Design review of the part built by this model. Coordinates are the model's own, in mm. A direction names the side the tool comes from. Coordinates: 2 decimals unless noted, no trailing zeros. Loops run counter-clockwise (first coordinate to the right, second up) from the corner with the lowest first, then second, coordinate; pieces in that order, holes last.
from build123d import *

# Parameters (mm, degrees)
SKETCH_2_R = 10


with BuildPart() as part:
    # 스윕1: sweep along a path in 스케치1
    with BuildLine(Plane.XY) as sweep_1_path:
        Line((0, 0), (60, 0))
        Line((60, 0), (60, 80))
        Line((60, 80), (110, 80))
        Line((110, 80), (110, -120))
        Line((110, -120), (30, -120))
        Line((30, -120), (30, -70))
    # 스케치2 → 스윕1 (sweep)
    with BuildSketch(Plane(origin=(0, 0, 0), x_dir=(0, 0, -1), z_dir=(1, 0, 0))):
        Circle(SKETCH_2_R)
    sweep(path=sweep_1_path.line, transition=Transition.RIGHT)


solid = part.part
Q1. Take a section at D-D, the plane x = 110. Write out the cut boundary in (y, z).
Q2. The part is to be moulded in two halves that separate along Y. For faces 4 (the flat face through (0, 0, 0)), 5 (the cylindrical face through (51.57, 40.7, -5.38)), say which applies: pulls with the +Y half, pulls with the -Y half, needs draft (parallel to the pull), parting line crosses it, or undercut.
Q3. For line 1 (Y direction, x = 38.5, z = -1); line 2 (Y direction, x = 64.5, z = 0.75); line 3 (X direction, y = -71.5, z = 7.5), list the stretches that pass through material, from the lowest coordinate up.
Q4. Machinability: for faces 1 (the cylindrical face through (69.3, -129.915, 1.302)), 2 (the cylindrical face through (27.71, -9.76, 2.17)), 3 (the flat face through (30, -70, 0)), which of the approach directions +Z, -Z, +X, -X, +Y, -Y give a long, thin tool a straight path to every point of the face, cutting with its end or side? Answer none if there is none.
Q5. Take a section at A-A, the plane x = 30. Write out the cut boundary in (y, z).
Q6. Take a section at C-C, the plane z = 0. Write out the cut boundary in (x, y).
Q7. Clearance check with flat-ended pins moving along their axes: pin 1 Ø10 at (x, z) = (25.5, 7) entering from -Y; pin 2 Ø6 at (y, z) = (-71.5, 0.5) entering from +X; pin 3 Ø10 at (x, z) = (28, 2.5) entering from +Y; pin 4 Ø10 at (x, z) = (91, -6) entering from -Y. State where each tip first meets the part, or that it passes through.
Q8. Take a section at B-B, the plane y = 60.5. Write out the cut boundary in (x, z), then the cut area to 3 significant figures.
Entries:
1. outline: (-120, -10) - (80, -10) arc R10 ccw to (80, 10) - (-120, 10) arc R10 ccw to start
2. face 4: needs draft
2. face 5: undercut
3. line 1: y = -129.95 to -70, -9.95 to 9.95
3. line 2: y = -129.97 to -110.03, -9.97 to 89.97
3. line 3: x = 23.39 to 36.61, 103.39 to 116.61
4. face 1: none
4. face 2: -X
4. face 3: +Z, -Z, -X
5. outline: (-120, -10) - (-70, -10) - (-70, 10) - (-120, 10) arc R10 ccw to start; circle Ø20 at (0, 0)
6. outline: (0, -10) - (70, -10) - (70, 70) - (100, 70) - (100, -110) - (40, -110) - (40, -70) - (20, -70) - (20, -130) - (120, -130) - (120, 90) - (50, 90) - (50, 10) - (0, 10) - close
7. pin 1: stops at y = -129.8
7. pin 2: stops at x = 120
7. pin 3: stops at y = 10
7. pin 4: stops at y = -129.95
8. outline: circle Ø20 at (60, 0); circle Ø20 at (110, 0)
8. area: 628 mm2
